Autodesk Inventor part; units mm, degrees
ref_plane "YZ Plane" through (0, 0, 0) normal (1, 0, 0) x (0, 1, 0)
ref_plane "XZ Plane" through (0, 0, 0) normal (0, 1, 0) x (-1, 0, 0)
ref_plane "XY Plane" through (0, 0, 0) normal (0, 0, 1) x (1, 0, 0)
sketch "Skizze1" plane through (0, 0, 0) normal (0, 0, 1) x (1, 0, 0)
  line L0 (0, 0) -> (0, 18)
  line L1 (8.5, 12.5) -> (24, 12.5)
  line L2 (46, 10) -> (46, 8.3)
  arc A0 (46, 8.3) -> (46.6, 7.7) centre (46.6, 8.3) ccw
  line L3 (46.6, 7.7) -> (47.9536, 7.7)
  arc A1 (47.9536, 7.7) -> (48.2536, 7.7804) centre (47.9536, 8.3) ccw
  line L4 (48.2536, 7.7804) -> (49.5, 8.5)
  line L5 (72.5, 3) -> (72.5, 0)
  line L6 (0, 0) -> (72.5, 0)
  line L7 (-14.5, 0) -> (87, 0) construction
  line L8 (32.5, 10) -> (46, 10)
  line L9 (60, 7.5) -> (60, 3)
  line L10 (60, 3) -> (72.5, 3)
  line L11 (49.5, 8.5) -> (59, 8.5)
  line L12 (60, 7.5) -> (59, 8.5)
  line L13 (64, -11.5) -> (64, 11.5) construction
  line L14 (0, 18) -> (8.5, 18)
  line L15 (8.5, 18) -> (8.5, 12.5)
  line L16 (24, 12.5) -> (24, 12.3)
  line L17 (32.5, 10) -> (32.5, 9.8)
  line L18 (32.5, 9.8) -> (28, 9.8)
  line L19 (28, 9.8) -> (28, 12.3)
  line L20 (28, 12.3) -> (24, 12.3)
  point P0 (60, 8.5)
  dimension "d0" = 25
  dimension "d3" = 0.6
  dimension "d4" = 0.6
  dimension "d7" = 3.5
  dimension "d35" = 15.4
  dimension "d36" = 24
  dimension "d37" = 32.5
  dimension "d38" = 20
  dimension "d39" = 46
  dimension "d40" = 17
  dimension "d41" = 30
  dimension "d42" = 1
  dimension "d43" = 1
  dimension "d44" = 60
  dimension "d45" = 6
  dimension "d56" = 8.5
  dimension "d57" = 36
  dimension "d58" = 8.5
  dimension "d60" = 0.2
  dimension "d61" = 0.2
  dimension "d62" = 4
revolve "Grundprofil" add sketch "Skizze1" angle 360 about axis through (-10, 0, 0) along (1, 0, 0)
sketch "Skizze2" plane through (0, 0, 0) normal (-1, 0, 0) x (0, 0, 1)
  point P0 (0, 0)
  point P1 (0, 0)
hole "M8 Sacklochbohrung" at (0, 0, 0) direction (1, 0, 0) diameter 6.647 depth 20 tip angle 118
thread "M17x1mm Aussenfeingewinde"
fillet "Kerbwirkungsreduktion 0.5mm" radius 0.5 1 edges at (60, -3, 0)
chamfer "Fase4" distance 0.5 angle 45 5 edges at (0, -18, 0) (8.5, -18, 0) (28, -12.3, 0) (46, -10, 0) (72.5, -3, 0)
properties part number "Shoulder_Shaft_Pitch" material "Stahl, hochfest, niedrig legiert"
Verification items for the finished model (mm, model axes). A direction names the side the tool comes from. Coordinates: 2 decimals unless noted, no trailing zeros. Write each loop counter-clockwise with the first axis right and the second up, starting at its lowest first coordinate (ties: lowest second). Pieces come first, ordered by that corner, then holes. Notation, with made-up numbers: (-18.75, -30.75) - (4.25, -30.75) arc R22 ccw to (4.25, 6.25) - close; hole circle Ø10 at (0.25, 36). An arc over 180 degrees is marked (long way). Answer as a JSON object with one key per item and string values.
(1) Cross-section at A-A on x = 29. Record the cut outline in (y, z).
Report:
{"outline": "circle Ø19.6 at (0, 0)"}
(2) Mould release check, pull along Z, two halves, no side actions. Record for faces 4 (the cylindrical face through (39.09, -2.17, -9.76)), 5 (the conical face through (21.65, 0.17, 0.55)), 6 (the flat face through (28, 2, 10)), 7 (the cylindrical face through (10.14, 1.27, 3.07)): pulls with the +Z half, pulls with the -Z half, needs draft (parallel to the pull), parting line crosses it, or undercut.
Report:
{"face 4": "parting line crosses it", "face 5": "undercut", "face 6": "needs draft", "face 7": "undercut"}
(3) Thickness scan on line 1 along Z through (x, y) = (6, 0); line 2 along Z through (x, y) = (12.5, 0); line 3 along X through (y, z) = (-2, -11). Record the ranges inside material, lowest first.
Report:
{"line 1": "-18 to -3.32, 3.32 to 18", "line 2": "-12.5 to -3.32, 3.32 to 12.5", "line 3": "0 to 28"}
(4) Gauge pin test, flat ends, axial feed: pin 1 Ø8 at (x, z) = (26.5, 1) entering from -Y; pin 2 Ø10 at (x, y) = (52, 8) entering from -Z; pin 3 Ø5 at (x, z) = (29.5, -5) entering from -Y. Record the tip position at first contact, or that the pin passes through.
Report:
{"pin 1": "y = -12.5", "pin 2": "z = -7.95", "pin 3": "y = -11.79"}
(5) Tool access check on faces 1 (the cylindrical face through (30.218, -2.124, 9.567)), 2 (the cylindrical face through (16.358, 11.923, 3.755)), 3 (the flat face through (0, 0, -4)). Record the directions out of +Z, -Z, +X, -X, +Y, -Y that give a thin tool (end or side, any length) a straight path to the whole face; none if there is none.
Report:
{"face 1": "none", "face 2": "+X", "face 3": "+Z, -Z, -X, +Y, -Y"}
(6) Cross-section at B-B on x = 10. Record the cut outline in (y, z), plus the area to 3 significant figures.
Report:
{"outline": "circle Ø25 at (0, 0); hole circle Ø6.65 at (0, 0)", "area": "456 mm^2"}
